Geometry check sheet. Reference: the model listing, model coordinates, mm. Face numbers are marked on the shaded views. A direction names the side the tool comes from. Give positions to 0.01 mm unless a question says otherwise; leave off trailing zeros. Order: outer loops, then holes, each group sorted by start corner. A loop starts at its lowest first (then second) coordinate and runs counter-clockwise, first axis right, second up. Notation, with made-up numbers: M -31,59.25 L -6,59.25 A21 cw -6,85.25 Z; hole C 32,-27.5 d5. An arc over 180 degrees is marked long. One line per question, with ' | ' between items. Start each with the question number.
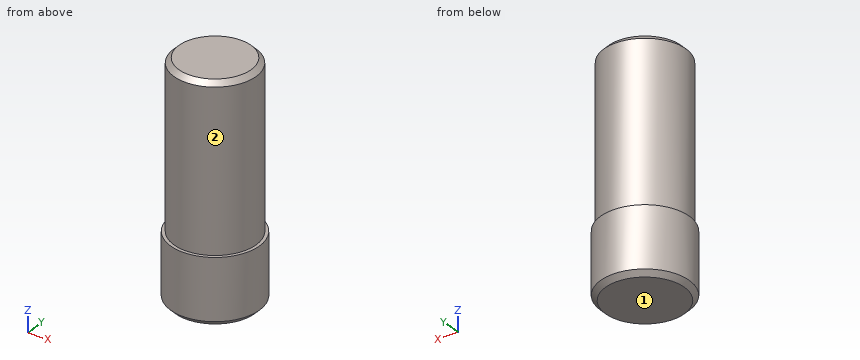
Autodesk Inventor part; units mm, degrees
ref_plane "YZ Plane" through (0, 0, 0) normal (1, 0, 0) x (0, 1, 0)
ref_plane "XZ Plane" through (0, 0, 0) normal (0, 1, 0) x (-1, 0, 0)
ref_plane "XY Plane" through (0, 0, 0) normal (0, 0, 1) x (1, 0, 0)
sketch "Sketch1" plane through (0, 0, 0) normal (0, 0, 1) x (1, 0, 0)
  circle A0 centre (-34.8653, 6.0523) radius 3.429
  circle A1 centre (-34.8653, 6.0523) radius 3.429
  dimension "d0" = 6.858
extrude "Extrusion1" add sketch "Sketch1" against normal blind 5.08
chamfer "Chamfer1" distance 0.381 angle 45 1 edges at (-38.2943, 6.0523, -5.08)
sketch "Sketch2" plane through (-34.8653, 6.0523, 0) normal (0, 0, 1) x (1, 0, 0)
  circle A0 centre (0, 0) radius 3.429
  circle A1 centre (0, 0) radius 3.175
  dimension "d5" = 6.35
extrude "Extrusion2" add sketch "Sketch2" along normal blind 12.7 contours A1
chamfer "Chamfer2" distance 0.381 angle 45 1 edges at (-38.0403, 6.0523, 12.7)
thread "Thread1"
properties part number "BUSS-STUD-250X50" material "Steel, High Strength Low Alloy"
Item 1: Set-up check for the marked faces 1 and 2: record each of +Z, -Z, +X, -X, +Y, -Y from which the full face is reachable in a straight line by a thin tool's end or side.
Item 2: Cross-section at A-A, the plane z = -2. Record the cut outline in (x, y), plus the area to 3 significant figures.
Item 3: Cross-section at B-B, the plane z = 11. Record the cut outline in (x, y) (3 decimals).
Item 4: Depth check by flat-ended pin: pin 1 (2 mm diameter, centred on x = -34.5, z = 6, fed in from +Y); pin 2 (1 mm diameter, centred on y = 7, z = 6.5, fed in from +X); pin 3 (4 mm diameter, centred on x = -37.5, z = -2, fed in from -Y). Enter the tip coordinate at first touch or a pass-through.
Item 5: Material ranges on line 1 along Y through (x, z) = (-35, 11.5); line 2 along Y through (x, z) = (-35, -4.5); line 3 along X through (y, z) = (6, 1), recorded low to high.
Outcome:
1) face 1: -Z, +X, -X, +Y, -Y | face 2: +Z
2) outline: C -34.87,6.05 d6.86 | area: 36.9 mm²
3) outline: C -34.865,6.052 d6.35
4) pin 1: stops at y = 9.23 | pin 2: stops at x = -31.72 | pin 3: stops at y = 2.68
5) line 1: y = 2.88 to 9.22 | line 2: y = 2.63 to 9.48 | line 3: x = -38.04 to -31.69
